CAD build for the part. Positions are in the model's coordinates, mm. A direction names the side the tool comes from. Round coordinates to 2 decimals unless told otherwise and drop trailing zeros. Loops run counter-clockwise (first coordinate to the right, second up) from the corner with the lowest first, then second, coordinate; pieces in that order, holes last.
```python
from build123d import *

# Parameters (mm, degrees)
F0_W     = 100
F0_H     = 100
F1_DEPTH = 50
F2_R     = 25
F3_DEPTH = 30
F5_DEPTH = 25.4


with BuildPart() as f1:
    # F0 (on Front) → F1 (new body)
    with BuildSketch(Plane.XZ):
        Rectangle(F0_W, F0_H)
    extrude(amount=F1_DEPTH)

    # F2 (on face) → F3 (join)
    with BuildSketch(Plane.XZ.offset(50)):
        Circle(F2_R)
    extrude(amount=F3_DEPTH)

    # F4 (on face) → F5 (join)
    with BuildSketch(Plane.XZ.offset(50)):
        Polygon((45.773503, 19.977803), (42.905975, 24.988901), (37.132472, 25.011099), (34.226497, 20.022197), (37.094025, 15.011099), (42.867528, 14.988901), align=None)
    extrude(amount=F5_DEPTH)


solid = f1.part
```
Item 1: 3-axis set-ups, long thin cutter, end or side, ignore diameter. For faces 1 (the flat face through (35.7, -62.52, 22.55)), 2 (the flat face through (44.36, -62.52, 22.45)), 3 (the flat face through (40, -75.4, 20)), 4 (the flat face through (-23, -50, 12)): which of +Z, -Z, +X, -X, +Y, -Y reach the whole face in a straight line?
Answers follow:
face 1: +Z, -Y
face 2: +Z, +X, -Y
face 3: +Z, -Z, +X, -Y
face 4: -Y
Item 2: Cut at D-D, the plane x = -29. Give the cut face in (y, z), plus the area to 3 significant figures.
Answers follow:
outline: (-50, -50) - (0, -50) - (0, 50) - (-50, 50) - close
area: 5,000 mm2
Item 3: Cut at A-A, the plane y = -73. Give the cut face in (x, z), plus the area to 3 significant figures.
Answers follow:
outline: circle Ø50 at (0, 0); (34.23, 20.02) - (37.09, 15.01) - (42.87, 14.99) - (45.77, 19.98) - (42.91, 24.99) - (37.13, 25.01) - close
area: 2,050 mm2
Item 4: Cut at B-B, the plane z = 0. Give the cut face in (x, y), plus the area to 3 significant figures.
Answers follow:
outline: (-50, -50) - (-25, -50) - (-25, -80) - (25, -80) - (25, -50) - (50, -50) - (50, 0) - (-50, 0) - close
area: 6,500 mm2
Item 5: Probe line 1 (Y direction, x = 39, z = 7); line 2 (Y direction, x = 37.5, z = 15.5); line 3 (X direction, y = -62, z = -10.5). List the from-to ranges inside material, lowest first.
Answers follow:
line 1: y = -50 to 0
line 2: y = -75.4 to 0
line 3: x = -22.69 to 22.69
Item 6: Cut at C-C, the plane x = 0. Give the cut face in (y, z), plus the area to 3 significant figures.
Answers follow:
outline: (-80, -25) - (-50, -25) - (-50, -50) - (0, -50) - (0, 50) - (-50, 50) - (-50, 25) - (-80, 25) - close
area: 6,500 mm2
Item 7: Flat gauge pins, fed straight in: P1, Ø10, axis at x = 19, z = 30, coming from the -Y side; P2, Ø10, axis at y = -56.5, z = -7.5, coming from the +X side; P3, Ø10, axis at y = -59.5, z = -6, coming from the -X side. Where does each tip first touch, or does it go through?
Answers follow:
P1: stops at y = -50
P2: stops at x = 24.87
P3: stops at x = -24.98
